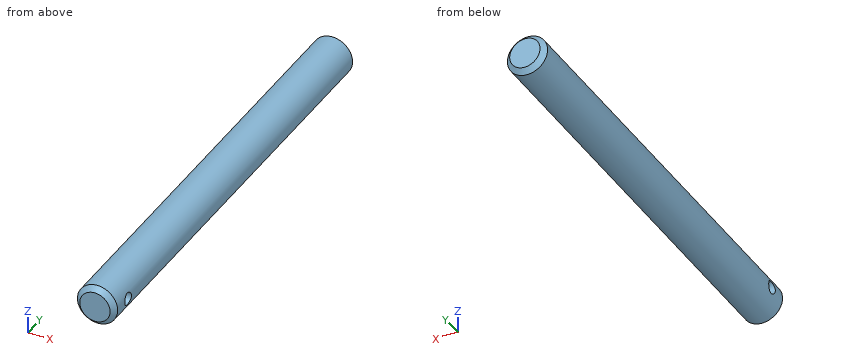
Autodesk Inventor part; units mm, degrees
ref_plane "Arbeitsebene1" through (3.25, 0, 0) normal (1, 0, 0) x (0, 1, 0)
ref_plane "XZ Plane" through (0, 0, 0) normal (0, 1, 0) x (-1, 0, 0)
ref_plane "XY Plane" through (0, 0, 0) normal (0, 0, 1) x (1, 0, 0)
sketch "Skizze1" plane through (0, 0, 0) normal (0, 1, 0) x (-1, 0, 0)
  circle A0 centre (0, 0) radius 3.25
  dimension "d0" = 6.5
extrude "Extrusion1" add sketch "Skizze1" along normal blind 73
chamfer "Fasen1" distance 0.8 angle 45 2 edges at (3.25, 73, 0) (3.25, 0, 0)
ref_plane "Arbeitsebene1" through (3.25, 0, 0) normal (1, 0, 0) x (0, 1, 0)
sketch "Skizze2" plane through (3.25, 0, 0) normal (1, 0, 0) x (0, 1, 0)
  point P0 (0, 0)
  point P1 (4, 0)
  dimension "d7" = 4
hole "Bohrung1" at (3.25, 4, 0) direction (-1, 0, 0) diameter 2 end through all
properties part number "BMS_fiiting_long" material "Edelstahl"
Verification items for the finished model (mm, model axes). Coordinates: 2 decimals unless noted, no trailing zeros. Order: outer loops, then holes, each group sorted by start corner. A loop starts at its lowest first (then second) coordinate and runs counter-clockwise, first axis right, second up. Notation, with made-up numbers: (-38, -34) -> (-10, -34) arc R20 ccw to (-10, -9) -> close; hole circle Ø1 at (-21, 34.25). An arc over 180 degrees is marked (long way). Answer as CSV lines item,"result". Start each with the question number.
1) Cross-section at A-A, the plane z = 0. Record the boundary of the cut face in (x, y), then the cut area to 3 significant figures.
2) Material ranges on L1, parallel to Z at x = -0.25, y = 4; L2, parallel to Y at x = 1, z = 0; L3, parallel to Z at x = -1.25, y = 4, recorded low to high. Write a range as [from, to].
3) Cross-section at C-C, the plane y = 4. Record the boundary of the cut face in (x, z).
4) Cross-section at B-B, the plane y = 42. Record the boundary of the cut face in (x, z).
5) Gauge pin test, flat ends, axial feed: pin 1 Ø1.8 at (y, z) = (4, 0) entering from -X; pin 2 Ø3 at (x, y) = (1, 62.5) entering from +Z. Record the tip position at first contact, or that the pin passes through.
Conclusion:
1,outline,"(-3.25, 0.8) -> (-2.45, 0) -> (2.45, 0) -> (3.25, 0.8) -> (3.25, 3) -> (-3.25, 3) -> close; (-3.25, 5) -> (3.25, 5) -> (3.25, 72.2) -> (2.45, 73) -> (-2.45, 73) -> (-3.25, 72.2) -> close"
1,area,"460 mm²"
2,L1,"z = [-3.24, -1], [1, 3.24]"
2,L2,"y = [0, 3], [5, 73]"
2,L3,"z = [-3, -1], [1, 3]"
3,outline,"(-3.09, -1) arc R3.25 ccw to (3.09, -1) -> close; (-3.09, 1) -> (3.09, 1) arc R3.25 ccw to start"
4,outline,"circle Ø6.5 at (0, 0)"
5,pin 1,"passes through"
5,pin 2,"stops at z = 3.25"
